from build123d import *

# Parameters (mm, degrees)
SKETCH1_W           = 149.86
SKETCH1_H           = 57.15
SKETCH1_W_2         = 19.05
SKETCH1_H_2         = 6.35
BOSS_EXTRUDE1_DEPTH = 6.35
SKETCH2_W           = 6.35
SKETCH2_H           = 9.525
SKETCH2_W_2         = 9.525
SKETCH2_H_2         = 6.35
BOSS_EXTRUDE2_DEPTH = 6.35


with BuildPart() as part:
    # Sketch1 → Boss-Extrude1 (new body)
    with BuildSketch(Plane(origin=(0, 0, 0), x_dir=(1, 0, 0), z_dir=(0, 1, 0))):
        with Locations((74.93, -28.575)):
            Rectangle(SKETCH1_W, SKETCH1_H)
        with Locations((15.875, -47.625)):
            Rectangle(SKETCH1_W_2, SKETCH1_H_2, mode=Mode.SUBTRACT)
        with Locations((15.875, -9.525)):
            Rectangle(SKETCH1_W_2, SKETCH1_H_2, mode=Mode.SUBTRACT)
        with Locations((133.985, -47.625)):
            Rectangle(SKETCH1_W_2, SKETCH1_H_2, mode=Mode.SUBTRACT)
        with Locations((133.985, -9.525)):
            Rectangle(SKETCH1_W_2, SKETCH1_H_2, mode=Mode.SUBTRACT)
    extrude(amount=BOSS_EXTRUDE1_DEPTH)

    # Sketch2 → Boss-Extrude2 (add)
    with BuildSketch(Plane.XZ):
        with Locations((-3.175, 14.2875)):
            Rectangle(SKETCH2_W, SKETCH2_H)
        with Locations((-3.175, 33.3375)):
            Rectangle(SKETCH2_W, SKETCH2_H)
        with Locations((-3.175, 52.3875)):
            Rectangle(SKETCH2_W, SKETCH2_H)
        with Locations((153.035, 14.4145)):
            Rectangle(SKETCH2_W, SKETCH2_H)
        with Locations((33.3375, 60.325)):
            Rectangle(SKETCH2_W_2, SKETCH2_H_2)
        with Locations((14.2875, 60.325)):
            Rectangle(SKETCH2_W_2, SKETCH2_H_2)
        with Locations((52.3875, 60.325)):
            Rectangle(SKETCH2_W_2, SKETCH2_H_2)
        with Locations((71.4375, 60.325)):
            Rectangle(SKETCH2_W_2, SKETCH2_H_2)
        with Locations((90.4875, 60.325)):
            Rectangle(SKETCH2_W_2, SKETCH2_H_2)
        with Locations((109.5375, 60.325)):
            Rectangle(SKETCH2_W_2, SKETCH2_H_2)
        with Locations((128.5875, 60.325)):
            Rectangle(SKETCH2_W_2, SKETCH2_H_2)
        Polygon((142.875, 63.5), (142.875, 57.15), (149.86, 57.15), (149.86, 47.752), (156.21, 47.752), (156.21, 57.277), (152.4, 57.277), (152.4, 63.5), align=None)
        with Locations((14.2875, -3.175)):
            Rectangle(SKETCH2_W_2, SKETCH2_H_2)
        with Locations((147.6375, -3.175)):
            Rectangle(SKETCH2_W_2, SKETCH2_H_2)
        with Locations((128.5875, -3.175)):
            Rectangle(SKETCH2_W_2, SKETCH2_H_2)
        with Locations((109.5375, -3.175)):
            Rectangle(SKETCH2_W_2, SKETCH2_H_2)
        with Locations((90.4875, -3.175)):
            Rectangle(SKETCH2_W_2, SKETCH2_H_2)
        with Locations((71.4375, -3.175)):
            Rectangle(SKETCH2_W_2, SKETCH2_H_2)
        with Locations((52.3875, -3.175)):
            Rectangle(SKETCH2_W_2, SKETCH2_H_2)
        with Locations((33.3375, -3.175)):
            Rectangle(SKETCH2_W_2, SKETCH2_H_2)
        with Locations((153.035, 33.4645)):
            Rectangle(SKETCH2_W, SKETCH2_H)
    extrude(amount=-BOSS_EXTRUDE2_DEPTH)


solid = part.part
Model file for the job. Use its own axes, mm. A direction names the side the tool comes from. Coordinates: 2 decimals unless noted, no trailing zeros. Write each loop counter-clockwise with the first axis right and the second up, starting at its lowest first coordinate (ties: lowest second). Pieces come first, ordered by that corner, then holes. Notation, with made-up numbers: (-16.5, -37) - (37.5, -37) arc R12 ccw to (37.5, -32) - close; hole circle Ø1 at (-11, 82.25). An arc over 180 degrees is marked (long way). Write each question's results on one line, items separated by ' | '. Start each with the question number.
1) Cut at D-D (x = 61). Write the cut outline in (y, z).
2) Cut at A-A (x = 131). Write the cut outline in (y, z).
3) Cut at C-C (y = 3.5). Count the separate pieces of the cut face and the enclosed holes in it, then the cut area to 3 significant figures.
4) Flat gauge pins, fed straight in: P1, Ø1.9, axis at y = 3.5, z = -4.5, coming from the -X side (3 decimals); P2, Ø1.9, axis at x = 62.5, y = 2, coming from the -Z side; P3, Ø1.9, axis at x = 154.5, y = 3.5, coming from the -Z side. Where does each tip first touch, or does it go through?
5) 3-axis set-ups, long thin cutter, end or side, ignore diameter. For faces 4 (the face through (57.15, 3, 60)), 5 (the face through (9.525, 3, -3)), 6 (the face through (104.775, 3, -3)), 7 (the face through (134, 3, 50.8)): which of +Z, -Z, +X, -X, +Y, -Y reach the whole face in a straight line?
6) Mould opens along Z. For faces 1 (the face through (43, 3, 0)), 2 (the face through (95.25, 3, 60)), 3 (the face through (-3, 3, 38.1)) say: pulls with the +Z half, pulls with the -Z half, needs draft (parallel to the pull), parting line crosses it, or undercut.
7) Cut at B-B (z = 8). Write the cut outline in (x, y).
8) Probe line 1 along X through (y, z) = (0.5, 46.5); line 2 along Z through (x, y) = (143, 5.5); line 3 along X through (y, z) = (1.5, 50). List the from-to ranges inside material, lowest first. Write a range as from..to.
Returned:
1) outline: (0, 0) - (6.35, 0) - (6.35, 57.15) - (0, 57.15) - close
2) outline: (0, -6.35) - (6.35, -6.35) - (6.35, 6.35) - (0, 6.35) - close; (0, 12.7) - (6.35, 12.7) - (6.35, 44.45) - (0, 44.45) - close; (0, 50.8) - (6.35, 50.8) - (6.35, 63.5) - (0, 63.5) - close
3) separate pieces: 1 | enclosed holes: 4 | area: 9,410 mm^2
4) P1: x = 9.525 | P2: z = 0 | P3: z = 9.65
5) face 4: +Z, +Y, -Y | face 5: -Z, -X, +Y, -Y | face 6: -Z, +Y, -Y | face 7: +Y, -Y
6) face 1: pulls with the -Z half | face 2: needs draft | face 3: undercut
7) outline: (0, 0) - (6.35, 0) - (6.35, 6.35) - (0, 6.35) - close; (25.4, 0) - (124.46, 0) - (124.46, 6.35) - (25.4, 6.35) - close; (143.51, 0) - (149.86, 0) - (149.86, 6.35) - (143.51, 6.35) - close
8) line 1: 0..6.35, 25.4..124.46, 143.51..149.86 | line 2: -6.35..6.35, 12.7..44.45, 50.8..63.5 | line 3: -6.35..6.35, 25.4..124.46, 143.51..156.21
